```python
from build123d import *

# Parameters (mm, degrees)
SKETCH1_W                   = 50.8
SKETCH1_H                   = 25.4
BOSS_EXTRUDE1_DEPTH         = 12.7
SKETCH2_W                   = 43
SKETCH2_H                   = 43
SKETCH2_R                   = 12.5
BOSS_EXTRUDE2_DEPTH         = 12.7
CHAMFER1_SIZE               = 12.7
TAP_DRILL_FOR_M3X0_5_TAP1_D = 2.5
F_1_4_CLEARANCE_HOLE1_D     = 6.7564
SKETCH8_R                   = 5.715
CUT_EXTRUDE1_DEPTH          = 7.112


with BuildPart() as part:
    # Sketch1 → Boss-Extrude1 (new body)
    with BuildSketch(Plane(origin=(0, 0, 0), x_dir=(1, 0, 0), z_dir=(0, 1, 0))):
        Rectangle(SKETCH1_W, SKETCH1_H)
    extrude(amount=BOSS_EXTRUDE1_DEPTH)

    # Sketch2 → Boss-Extrude2 (add)
    with BuildSketch(Plane.ZY.offset(25.4)):
        with Locations((0, 34.2)):
            Rectangle(SKETCH2_W, SKETCH2_H)
        with Locations((0, 34.2)):
            Circle(SKETCH2_R, mode=Mode.SUBTRACT)
    extrude(amount=-BOSS_EXTRUDE2_DEPTH)

    # Chamfer1
    # the kernel refuses this chamfer: 12.7 mm, written as the material it adds along each edge
    with BuildSketch(Plane(origin=(-25.4, 12.7, 12.7), x_dir=(0, -0.9996219169112966, -0.027495876610586334), z_dir=(1, 0, 0))) as chamfer1_piece_1_section:
        Polygon((CHAMFER1_SIZE * 0.999621916911, -CHAMFER1_SIZE * 0.0274958766106), (-CHAMFER1_SIZE * 0.0274958766106, -CHAMFER1_SIZE * 0.999621916911), (0, 0), align=None)
    chamfer1_piece_1 = extrude(amount=12.7, mode=Mode.PRIVATE)
    chamfer1_piece_1 = split(chamfer1_piece_1, bisect_by=Plane(origin=(-19.05, 8.16124498, 21.5), z_dir=(0, 0, -1)), keep=Keep.TOP, mode=Mode.PRIVATE)
    add(chamfer1_piece_1)
    with BuildSketch(Plane(origin=(-12.7, 12.7, -12.7), x_dir=(0, -0.9996219169112966, 0.027495876610586334), z_dir=(-1, 0, 0))) as chamfer1_piece_2_section:
        Polygon((CHAMFER1_SIZE * 0.999621916911, -CHAMFER1_SIZE * 0.0274958766106), (-CHAMFER1_SIZE * 0.0274958766106, -CHAMFER1_SIZE * 0.999621916911), (0, 0), align=None)
    chamfer1_piece_2 = extrude(amount=12.7, mode=Mode.PRIVATE)
    chamfer1_piece_2 = split(chamfer1_piece_2, bisect_by=Plane(origin=(-19.05, 8.16124498, -21.5), z_dir=(0, 0, 1)), keep=Keep.TOP, mode=Mode.PRIVATE)
    add(chamfer1_piece_2)

    # Tap Drill for M3x0.5 Tap1 (through all)
    with Locations(Plane.ZY.offset(25.4)):
        with Locations((-15.160825054, 49.7), (15.5, 49.7), (15.5, 18.7), (-15.5, 18.7)):
            Hole(TAP_DRILL_FOR_M3X0_5_TAP1_D / 2)

    # 1/4 Clearance Hole1 (through all)
    with Locations(Plane(origin=(0, 12.7, 0), x_dir=(1, 0, 0), z_dir=(0, 1, 0))):
        with Locations((-4.6, 0), (10.4, 0)):
            Hole(F_1_4_CLEARANCE_HOLE1_D / 2)

    # Sketch8 → Cut-Extrude1 (cut)
    with BuildSketch(Plane(origin=(0, 12.7, 0), x_dir=(1, 0, 0), z_dir=(0, 1, 0))):
        with Locations(Location((-4.6, 0, 0), (0, 0, 270))):
            Circle(SKETCH8_R)
        with Locations(Location((10.4, 0, 0), (0, 0, 270))):
            Circle(SKETCH8_R)
    extrude(amount=-CUT_EXTRUDE1_DEPTH, mode=Mode.SUBTRACT)


solid = part.part
```
Verification items for the finished model (mm, model axes). A direction names the side the tool comes from. Give positions to 0.01 mm unless a question says otherwise; leave off trailing zeros. Write each loop counter-clockwise with the first axis right and the second up, starting at its lowest first coordinate (ties: lowest second). Pieces come first, ordered by that corner, then holes. Notation, with made-up numbers: (32, -35.75) - (43, -35.75) arc R7 cw to (43, -28.75) - close; hole circle Ø9 at (-1, 39). An arc over 180 degrees is marked (long way). Put each result on its own line as item: value.
Q1. Section check A-A on y = 18.7. Record the cut outline in (x, z).
Result:
outline: (-25.4, -21.5) - (-12.7, -21.5) - (-12.7, -16.75) - (-25.4, -16.75) - close; (-25.4, -14.25) - (-12.7, -14.25) - (-12.7, 14.25) - (-25.4, 14.25) - close; (-25.4, 16.75) - (-12.7, 16.75) - (-12.7, 21.5) - (-25.4, 21.5) - close
Q2. Set-up check for faces 4 (the face through (6, 6, -12.7)), 5 (the face through (-19, 55.7, 0)), 6 (the face through (16.066, 9.194, -0.744)): record each of +Z, -Z, +X, -X, +Y, -Y from which the full face is reachable in a straight line by a thin tool's end or side.
Result:
face 4: -Z, +X, +Y, -Y
face 5: +Z, -Z, +X, -X, +Y
face 6: +Y
Q3. Section check D-D on y = 34.2. Record the cut outline in (x, z), and give its area (3 significant figures).
Result:
outline: (-25.4, -21.5) - (-12.7, -21.5) - (-12.7, -12.5) - (-25.4, -12.5) - close; (-25.4, 12.5) - (-12.7, 12.5) - (-12.7, 21.5) - (-25.4, 21.5) - close
area: 229 mm2
Q4. Depth check by flat-ended pin: P1, Ø4, axis at y = 42.5, z = 8, coming from the +X side; P2, Ø13, axis at y = 36, z = -4, coming from the +X side; P3, Ø1.5, axis at x = 4, y = 9, coming from the -Z side; P4, Ø3.5, axis at x = 10, z = -3, coming from the +Y side. Enter the tip coordinate at first touch or a pass-through.
Result:
P1: x = -12.7
P2: through
P3: z = -12.7
P4: y = 5.59
Q5. Section check B-B on z = 0. Record the cut outline in (x, y) (3 decimals).
Result:
outline: (-25.4, 0) - (-7.978, 0) - (-7.978, 5.588) - (-10.315, 5.588) - (-10.315, 12.7) - (-12.7, 12.7) - (-12.7, 21.7) - (-25.4, 21.7) - close; (-25.4, 46.7) - (-12.7, 46.7) - (-12.7, 55.7) - (-25.4, 55.7) - close; (-1.222, 0) - (7.022, 0) - (7.022, 5.588) - (4.685, 5.588) - (4.685, 12.7) - (1.115, 12.7) - (1.115, 5.588) - (-1.222, 5.588) - close; (13.778, 0) - (25.4, 0) - (25.4, 12.7) - (16.115, 12.7) - (16.115, 5.588) - (13.778, 5.588) - close
Q6. Mould release check, pull along Z, two halves, no side actions. Record for faces 1 (the face through (-19, 33, -21.5)), 2 (the face through (6, 6, 12.7)), 3 (the face through (-18.96, 48.48, 15.77)): released by +Z, released by -Z, zero draft, split by the parting line, or undercut.
Result:
face 1: released by -Z
face 2: released by +Z
face 3: undercut
Q7. Section check C-C on x = 10.4. Record the cut outline in (y, z) (3 decimals).
Result:
outline: (0, -12.7) - (12.7, -12.7) - (12.7, -5.715) - (5.588, -5.715) - (5.588, -3.378) - (0, -3.378) - close; (0, 3.378) - (5.588, 3.378) - (5.588, 5.715) - (12.7, 5.715) - (12.7, 12.7) - (0, 12.7) - close
Q8. Scan lines: probe 1 along X at (y, z) = (10, 0) (3 decimals); probe 2 along Z at (x, y) = (-17, 34); probe 3 along Y at (x, z) = (-19, 15). Record each from-to range of solid material in increasing order. Write a range as from..to.
Result:
probe 1: -25.4..-10.315, 1.115..4.685, 16.115..25.4
probe 2: -21.5..-12.5, 12.5..21.5
probe 3: 2.3..17.55, 19.85..48.55, 50.85..55.7
